Here's how the part is built. I have some questions about the finished solid (model axes, mm). A direction names the side the tool comes from. Coordinates: 2 decimals unless noted, no trailing zeros. Loops run counter-clockwise (first coordinate to the right, second up) from the corner with the lowest first, then second, coordinate; pieces in that order, holes last.
from build123d import *
from build123d.topology import SkipClean

# Parameters (mm, degrees)
SKETCH1_R                = 1.5
BOSS_EXTRUDE1_DEPTH      = 2.5
BOSS_EXTRUDE2_DEPTH      = 6.9
BOSS_EXTRUDE2_DEPTH_BACK = 2.5
SKETCH2_R                = 4.5
SKETCH2_R_2              = 1.5
SKETCH4_R                = 2.5
CUT_EXTRUDE1_DEPTH       = 2
BOSS_EXTRUDE3_START      = 0.75
SKETCH5_R                = 4.5
SKETCH5_R_2              = 2.5
BOSS_EXTRUDE3_DEPTH      = 0.75
BOSS_EXTRUDE4_DEPTH      = 2.5
CUT_EXTRUDE2_REACH       = 80.314
SKETCH7_W                = 7
SKETCH7_H                = 16.5
SKETCH7_W_2              = 16
SKETCH7_H_2              = 8
CUT_EXTRUDE3_REACH       = 82.041
SKETCH9_W                = 2.5
SKETCH9_H                = 22.388822383
BOSS_EXTRUDE5_DEPTH      = 12.5
FILLET2_R                = 1
FILLET3_R                = 4
CUT_EXTRUDE4_DEPTH       = 74.103052287
CUT_EXTRUDE4_DEPTH_BACK  = 74.103052287
SKETCH10_W               = 78.235731334
SKETCH10_H               = 6.290045588
SKETCH11_W               = 14.64
SKETCH11_H               = 2.5
BOSS_EXTRUDE6_DEPTH      = 12.5
BOSS_EXTRUDE7_DEPTH      = 2.5
SKETCH14_R               = 1.5
CUT_EXTRUDE5_DEPTH       = 2.5


with BuildPart() as part:
    # Sketch1 → Boss-Extrude1 (new body)
    with BuildSketch(Plane(origin=(0, 0, 0), x_dir=(0, 0, -1), z_dir=(1, 0, 0))):
        with BuildLine():
            Line((0, 12.5), (34.45, 12.5))
            Line((34.45, 12.5), (34.45, -12.5))
            Line((34.45, -12.5), (0, -12.5))
            ThreePointArc((0, -12.5), (-12.5, 0), (0, 12.5))
        make_face()
        Circle(SKETCH1_R, mode=Mode.SUBTRACT)
    extrude(amount=BOSS_EXTRUDE1_DEPTH)

    # Sketch2 → Boss-Extrude2 (add, two sides: drawn at the far end of the back side and taken through both)
    with BuildSketch(Plane.ZY.offset(-BOSS_EXTRUDE2_DEPTH_BACK)):
        Circle(SKETCH2_R)
        Circle(SKETCH2_R_2, mode=Mode.SUBTRACT)
    extrude(amount=BOSS_EXTRUDE2_DEPTH + BOSS_EXTRUDE2_DEPTH_BACK)

    # Sketch4 → Cut-Extrude1 (cut)
    with BuildSketch(Plane(origin=(2.5, 0, 0), x_dir=(0, 0, -1), z_dir=(1, 0, 0))):
        Circle(SKETCH4_R)
    extrude(amount=-CUT_EXTRUDE1_DEPTH, mode=Mode.SUBTRACT)

    # Sketch5 → Boss-Extrude3 (add)
    with SkipClean():  # the faces are left unmerged after this step: merging them gives an invalid solid
        with BuildSketch(Plane(origin=(2.5, 0, 0), x_dir=(0, 0, -1), z_dir=(1, 0, 0)).offset(BOSS_EXTRUDE3_START)):
            with Locations(Location((0, 0, 0), (0, 0, 180))):
                Circle(SKETCH5_R)
            Circle(SKETCH5_R_2, mode=Mode.SUBTRACT)
        extrude(amount=-BOSS_EXTRUDE3_DEPTH)

    # Sketch6 → Boss-Extrude4 (add)
    with SkipClean():  # the faces are left unmerged after this step: merging them gives an invalid solid
        with BuildSketch(Plane(origin=(0, 0, -34.45), x_dir=(-1, 0, 0), z_dir=(0, 0, -1))):
            Polygon((-8.812505246, 36.25), (53.321583376, 36.25), (53.321583376, -36.25), (6.25, -36.25), (-19.178416624, -36.25), (-19.178416624, 36.25), align=None)
        extrude(amount=-BOSS_EXTRUDE4_DEPTH)
    add(part.part.scale(1), mode=Mode.REPLACE)  # the faces are merged on a copy

    # Sketch7 → Cut-Extrude2 (cut, up to next)
    with BuildSketch(Plane.XY.offset(-31.95), mode=Mode.PRIVATE) as cut_extrude2_sk1:
        with Locations((-1.711858899, -11.632438111)):
            Rectangle(SKETCH7_W, SKETCH7_H)
    cut_extrude2_tool1 = extrude(cut_extrude2_sk1.sketch, amount=-CUT_EXTRUDE2_REACH, mode=Mode.PRIVATE) & part.part
    # Sketch7 → Cut-Extrude2 (cut, up to next)
    with BuildSketch(Plane.XY.offset(-31.95), mode=Mode.PRIVATE) as cut_extrude2_sk2:
        with Locations((-16.5, 0)):
            Rectangle(SKETCH7_W_2, SKETCH7_H_2)
    cut_extrude2_tool2 = extrude(cut_extrude2_sk2.sketch, amount=-CUT_EXTRUDE2_REACH, mode=Mode.PRIVATE) & part.part
    add(cut_extrude2_tool1.solids().sort_by_distance((-1.711859, -11.632438, -31.95))[0], mode=Mode.SUBTRACT)
    add(cut_extrude2_tool2.solids().sort_by_distance((-16.5, 0, -31.95))[0], mode=Mode.SUBTRACT)

    # Sketch9 → Cut-Extrude3 (cut, up to next)
    with BuildSketch(Plane.XZ.offset(12.5), mode=Mode.PRIVATE) as cut_extrude3_sk1:
        with Locations((1.25, -20.755588809)):
            Rectangle(SKETCH9_W, SKETCH9_H)
    cut_extrude3_tool1 = extrude(cut_extrude3_sk1.sketch, amount=-CUT_EXTRUDE3_REACH, mode=Mode.PRIVATE) & part.part
    add(cut_extrude3_tool1.solids().sort_by_distance((1.25, -12.5, -20.755589))[0], mode=Mode.SUBTRACT)


with BuildPart() as cut_extrude3_piece_1:
    # of the separate pieces the step leaves, piece 1, a body of its own (cut_extrude3_pieces)
    add(part.part.solids().sort_by_distance((-53.321583376, 36.25, -31.95))[0])



with BuildPart() as cut_extrude3_piece_2:
    # of the separate pieces the step leaves, piece 2, a body of its own (cut_extrude3_pieces)
    add(part.part.solids().sort_by_distance((0, 12.5, 0))[0])


with BuildPart() as cut_extrude3_piece_1_1:
    add(cut_extrude3_piece_1.part)

    add(cut_extrude3_piece_2.part)  # Boss-Extrude5 merges Cut-Extrude3 piece 2
    # Sketch8 → Boss-Extrude5 (add, symmetric)
    with BuildSketch(Plane(origin=(0, 0, 0), x_dir=(1, 0, 0), z_dir=(0, 1, 0))):
        with BuildLine():
            Line((0, 7.729605828), (2.5, 7.729605828))
            Line((2.5, 7.729605828), (2.5, 10.229605828))
            ThreePointArc((2.5, 10.229605828), (1.573627862, 16.099871922), (-1.115452176, 21.399592472))
            ThreePointArc((-1.115452176, 21.399592472), (-3.053519862, 25.219195088), (-3.721172696, 29.45))
            Line((-3.721172696, 29.45), (-3.721172696, 31.95))
            Line((-3.721172696, 31.95), (-6.221172696, 31.95))
            Line((-6.221172696, 31.95), (-6.221172696, 28.45))
            ThreePointArc((-6.221172696, 28.45), (-5.429444077, 23.92831405), (-3.148463103, 19.944646916))
            ThreePointArc((-3.148463103, 19.944646916), (-0.81124762, 15.862767844), (0, 11.229605828))
            Line((0, 11.229605828), (0, 7.729605828))
        make_face()
    extrude(amount=BOSS_EXTRUDE5_DEPTH, both=True)

    # Fillet2
    fillet2_edges = [cut_extrude3_piece_1_1.edges().sort_by_distance(p)[0] for p in [
        (-8.5, 4, -33.2),
        (-8.5, -4, -33.2),
        (-24.5, -4, -33.2),
        (-24.5, 4, -33.2),
        (-5.211858899, -19.882438111, -33.2),
        (-5.211858899, -3.382438111, -33.2),
        (1.788141101, -3.382438111, -33.2),
        (1.788141101, -19.882438111, -33.2),
    ]]
    fillet(fillet2_edges, radius=FILLET2_R)

    # Fillet3
    fillet3_edges = [cut_extrude3_piece_1_1.edges().sort_by_distance(p)[0] for p in [
        (19.178416624, 36.25, -33.2),
        (-53.321583376, 36.25, -33.2),
        (-53.321583376, -36.25, -33.2),
        (19.178416624, -36.25, -33.2),
    ]]
    fillet(fillet3_edges, radius=FILLET3_R)

    # Sketch10 → Cut-Extrude4 (cut, two sides: drawn at the far end of the back side and taken through both)
    with SkipClean():  # the faces are left unmerged after this step: merging them gives an invalid solid
        with BuildSketch(Plane(origin=(0, 0, 0), x_dir=(1, 0, 0), z_dir=(0, 1, 0)).offset(-CUT_EXTRUDE4_DEPTH_BACK)):
            with Locations((-17.391929865, 35.095022794)):
                Rectangle(SKETCH10_W, SKETCH10_H)
        extrude(amount=CUT_EXTRUDE4_DEPTH + CUT_EXTRUDE4_DEPTH_BACK, mode=Mode.SUBTRACT)

    # Sketch11 → Boss-Extrude6 (add, symmetric)
    with BuildSketch(Plane(origin=(0, 0, 0), x_dir=(1, 0, 0), z_dir=(0, 1, 0))):
        with Locations((3.598827304, 30.7)):
            Rectangle(SKETCH11_W, SKETCH11_H)
    boss_extrude6 = extrude(amount=BOSS_EXTRUDE6_DEPTH, both=True)

    # Sketch13 → Boss-Extrude7 (add)
    with BuildSketch(Plane(origin=(0, 0, -31.95), x_dir=(-1, 0, 0), z_dir=(0, 0, -1))):
        with BuildLine():
            Line((-10.918827304, 12.5), (4.081172696, 12.5))
            Line((4.081172696, 12.5), (4.081172696, 28.75))
            Line((4.081172696, 28.75), (4.081172696, 36.25))
            Line((4.081172696, 36.25), (-3.678827304, 36.25))
            Line((-3.678827304, 36.25), (-6.918827304, 36.25))
            ThreePointArc((-6.918827304, 36.25), (-9.747254429, 35.078427125), (-10.918827304, 32.25))
            Line((-10.918827304, 32.25), (-10.918827304, 28.75))
            Line((-10.918827304, 28.75), (-10.918827304, 12.5))
        make_face()
    boss_extrude7 = extrude(amount=-BOSS_EXTRUDE7_DEPTH)

    # Mirror1: Boss-Extrude6, Boss-Extrude7 across plane
    add(boss_extrude6.mirror(Plane.ZX))
    add(boss_extrude7.mirror(Plane.ZX))

    # Sketch14 → Cut-Extrude5 (cut)
    with BuildSketch(Plane(origin=(0, 0, -31.95), x_dir=(-1, 0, 0), z_dir=(0, 0, -1))):
        with Locations((-3.418827304, 28.75)):
            Circle(SKETCH14_R)
    cut_extrude5 = extrude(amount=-CUT_EXTRUDE5_DEPTH, mode=Mode.SUBTRACT)

    # Mirror2: Cut-Extrude5 across plane
    add(cut_extrude5.mirror(Plane.ZX), mode=Mode.SUBTRACT)


solid = cut_extrude3_piece_1_1.part
Q1. Suppose I cut it at D-D on z = -8. Write out the boundary of the cut face in (x, y).
Q2. Will these pins go through, and if not, where does the flat tip stop? P1, Ø25, axis at y = -5.5, z = -1, coming from the +X side; P2, Ø0.8, axis at y = -22.5, z = -31, coming from the -X side; P3, Ø8, axis at y = -14, z = -5, coming from the -X side; P4, Ø2.5, axis at x = -2.5, z = -10, coming from the +Y side.
Q3. Suppose I cut it at C-C on y = -7.5. Write out the boundary of the cut face in (x, z), and give its area (3 significant figures).
Q4. For faces 1 (the cylindrical face through (-5.45, 0.18, -23.99)), 2 (the cylindrical face through (-3.035, 0.175, -25.162)), 3 (the flat face through (-4.081, -24, -31)), 4 (the cylindrical face through (1.89, -2.44, 0.54)), which set-ups out of +Z, -Z, +X, -X, +Y, -Y let a thin tool reach every point of the face, with its end or its side?
Q5. Please list where these lines run through material, in increasing order: probe 1 along Y at (x, z) = (-1.5, 0); probe 2 along Z at (x, y) = (-1, -2); probe 3 along Z at (x, y) = (1, -23).
Q6. Suppose I cut it at B-B on x = -2. Write out the boundary of the cut face in (y, z).
Q7. We'd pull the mould along Y, two halves only. Please class faces 5 (the cylindrical face through (1.232, -0.275, 12.497)), 6 (the flat face through (0.5, -2, 0)), 7 (the cylindrical face through (3.614, 30.237, -30.718)), 8 (the cylindrical face through (-0.83, 0.18, -15.92)): pulls with the +Y half, pulls with the -Y half, needs draft (parallel to the pull), parting line crosses it, or undercut.
Q8. Suppose I cut it at A-A on y = -28.75. Write out the boundary of the cut face in (x, z), and give its area (3 significant figures).
Check values:
1. outline: (0, -12.5) - (2.5, -12.5) - (2.5, 12.5) - (0, 12.5) - close
2. P1: stops at x = 3.25
2. P2: stops at x = -4.08
2. P3: stops at x = 0
2. P4: passes through
3. outline: (-6.22, -31.95) - (10.92, -31.95) - (10.92, -29.45) - (-3.72, -29.45) arc R13.74 cw to (-1.12, -21.4) arc R19.06 ccw to (2.5, -10.23) - (2.5, 10) - (0, 10) - (0, -11.23) arc R13.64 cw to (-3.15, -19.94) arc R13.31 ccw to (-6.22, -28.45) - close
3. area: 145 mm2
4. face 1: -X, +Y, -Y
4. face 2: +X, +Y, -Y
4. face 3: +Z, -Z, -X, -Y
4. face 4: +X
5. probe 1: y = -4.5 to -1.5, 1.5 to 4.5
5. probe 2: z = -31.95 to -29.45, -21.24 to -16.36, -4.03 to 4.03
5. probe 3: z = -31.95 to -29.45
6. outline: (-36.25, -31.95) - (36.25, -31.95) - (36.25, -29.45) - (-36.25, -29.45) - close; (-12.5, -22.79) - (12.5, -22.79) - (12.5, -18.34) - (-12.5, -18.34) - close; circle Ø9 at (0, 0); hole circle Ø3 at (0, 0)
7. face 5: parting line crosses it
7. face 6: undercut
7. face 7: undercut
7. face 8: needs draft
8. outline: (-4.08, -31.95) - (1.92, -31.95) - (1.92, -29.45) - (-4.08, -29.45) - close; (4.92, -31.95) - (10.92, -31.95) - (10.92, -29.45) - (4.92, -29.45) - close
8. area: 30.0 mm2
